Here's how the part is built. I have some questions about the finished solid (model axes, mm). Give positions to 0.01 mm unless a question says otherwise; leave off trailing zeros. Loops run counter-clockwise (first coordinate to the right, second up) from the corner with the lowest first, then second, coordinate; pieces in that order, holes last.
Q1. We'd pull the mould along Z, two halves only. Please class faces 1 (the face through (20, 50, -50)), 2 (the face through (10, 50, -142)), 3 (the face through (3, 50, -46)): +Z half, -Z half, draft (parallel to the pull), parting line (faces both ways), or undercut.
Q2. If we section it at A-A (y = 30): Please give me the cut outline in (x, z), plus the area to 3 significant figures.
Q3. Will this pin go through, and if not, where does the flat tip stop? P1, Ø8, axis at y = 96.5, z = -48.5, coming from the -X side.
Q4. I need wall thicknesses on line 1 (Z direction, x = 1.5, y = 8); line 2 (X direction, y = 15, z = -87.5). Which ranges of each line are inside material? Lowest first, please.
Q5. If we section it at B-B (z = -21.5): Please give me the cut outline in (x, y).
from build123d import *

# Parameters (mm, degrees)
F0_W     = 182
F0_H     = 182
F0_W_2   = 102
F0_H_2   = 102
F1_DEPTH = 20
F2_DEPTH = 3
F3_W     = 11
F3_H     = 40
F4_DEPTH = 3


with BuildPart() as f1:
    # F0 (on Right) → F1 (new body)
    with BuildSketch(Plane.YZ):
        with Locations((51, -51)):
            Rectangle(F0_W, F0_H)
        with Locations((51, -51)):
            Rectangle(F0_W_2, F0_H_2, mode=Mode.SUBTRACT)
        with Locations((51, -51)):
            Rectangle(F0_W_2, F0_H_2)
    extrude(amount=F1_DEPTH)

    # F0 (on Right) → F2 (cut)
    with BuildSketch(Plane.YZ):
        with Locations((51, -51)):
            Rectangle(F0_W_2, F0_H_2)
    extrude(amount=F2_DEPTH, mode=Mode.SUBTRACT)

    # F3 (on face) → F4 (cut)
    with BuildSketch(Plane.YZ):
        with Locations((50.5, 20)):
            Rectangle(F3_W, F3_H)
    extrude(amount=F4_DEPTH, mode=Mode.SUBTRACT)


solid = f1.part
Check sheet entries:
1. face 1: draft
1. face 2: -Z half
1. face 3: undercut
2. outline: (0, -142) - (20, -142) - (20, 40) - (0, 40) - (0, 0) - (3, 0) - (3, -102) - (0, -102) - close
2. area: 3,330 mm2
3. P1: stops at x = 3
4. line 1: z = -142 to -102, 0 to 40
4. line 2: x = 3 to 20
5. outline: (0, -40) - (20, -40) - (20, 142) - (0, 142) - (0, 102) - (3, 102) - (3, 0) - (0, 0) - close
